Source: CAD feature listing. Evaluate the final solid. Frame: model axes, mm. Face numbers are marked on the shaded views. A direction names the side the tool comes from. Give positions to 0.01 mm unless a question says otherwise; leave off trailing zeros.
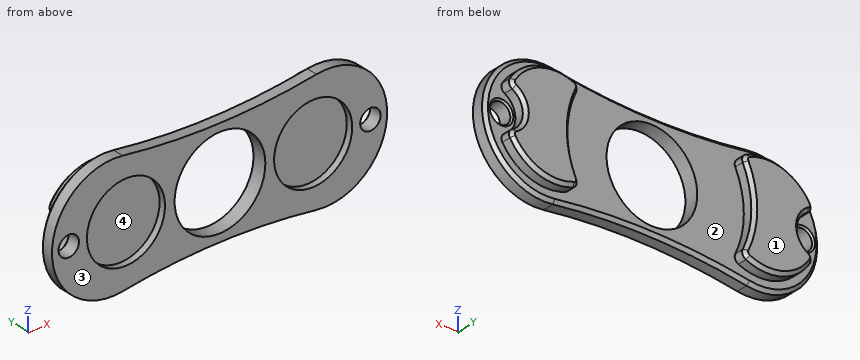
from build123d import *

# Parameters (mm, degrees)
F0_R      = 11.1
F1_DEPTH  = 7
F2_SIZE   = 0.8
F3_R      = 12.5
F4_DEPTH  = 3
F5_R      = 12.5
F6_DEPTH  = 3
F8_R      = 22.5
F9_DEPTH  = 3
F10_R     = 22.5
F11_DEPTH = 3
F12_R     = 5
F13_DEPTH = 3
F14_R     = 5
F15_DEPTH = 3
F16_R     = 5
F17_DEPTH = 3
F18_R     = 5
F19_DEPTH = 3
F20_R     = 1.5
F21_R     = 2.5
F22_DEPTH = 25
F23_R     = 2.5
F24_DEPTH = 25
F25_SIZE  = 0.4
F26_SIZE  = 0.8
F27_W     = 103.2572649419
F27_H     = 49.3412911892
F28_DEPTH = 6.5
F29_R     = 9.55
F30_DEPTH = 1.6


with BuildPart() as f1:
    # F0 (on Front) → F1 (new body)
    with BuildSketch(Plane.XZ):
        with BuildLine():
            ThreePointArc((21.7678643686, 14.8235294118), (-1.9380179843, 13), (-25.6439003372, 14.8235294118))
            ThreePointArc((-25.6439003372, 14.8235294118), (-42.9380179843, 0), (-25.6439003372, -14.8235294118))
            ThreePointArc((-25.6439003372, -14.8235294118), (-1.9380179843, -13), (21.7678643686, -14.8235294118))
            ThreePointArc((21.7678643686, -14.8235294118), (39.0619820157, 0), (21.7678643686, 14.8235294118))
        make_face()
        with Locations((-1.8380179843, 0)):
            Circle(F0_R, mode=Mode.SUBTRACT)
    extrude(amount=F1_DEPTH)

    # F2
    f2_edges = [f1.edges().sort_by_distance(p)[0] for p in [
        (-42.938018, -7, 0),
        (-1.938018, -7, -13),
        (-1.938018, 0, -13),
    ]]
    chamfer(f2_edges, length=F2_SIZE)

    # F3 (on face) → F4 (join)
    with BuildSketch(Plane.XZ.offset(7)):
        with Locations((-27.9380179843, 0)):
            Circle(F3_R)
        with Locations((24.0619820157, 0)):
            Circle(F3_R)
    extrude(amount=F4_DEPTH)

    # F5 (on face) → F6 (join)
    with BuildSketch(Plane(origin=(0, 0, 0), x_dir=(-1, 0, 0), z_dir=(0, 1, 0))):
        with Locations((-24.0619820157, 0)):
            Circle(F5_R)
        with Locations((27.9380179843, 0)):
            Circle(F5_R)
    extrude(amount=F6_DEPTH)

    # F8 (on face) → F9 (cut)
    with BuildSketch(Plane.XZ.offset(10)):
        with Locations((-1.8380179843, 0)):
            Circle(F8_R)
    extrude(amount=-F9_DEPTH, mode=Mode.SUBTRACT)

    # F10 (on face) → F11 (cut)
    with BuildSketch(Plane(origin=(0, 3, 0), x_dir=(-1, 0, 0), z_dir=(0, 1, 0))):
        with Locations((1.8380179843, 0)):
            Circle(F10_R)
    extrude(amount=-F11_DEPTH, mode=Mode.SUBTRACT)

    # F12 (on face) → F13 (cut)
    with BuildSketch(Plane(origin=(0, 3, 0), x_dir=(-1, 0, 0), z_dir=(0, 1, 0))):
        with Locations((-36.5619820157, 0)):
            Circle(F12_R)
    extrude(amount=-F13_DEPTH, mode=Mode.SUBTRACT)

    # F14 (on face) → F15 (cut)
    with BuildSketch(Plane(origin=(0, 3, 0), x_dir=(-1, 0, 0), z_dir=(0, 1, 0))):
        with Locations((40.4380179843, 0)):
            Circle(F14_R)
    extrude(amount=-F15_DEPTH, mode=Mode.SUBTRACT)

    # F16 (on face) → F17 (cut)
    with BuildSketch(Plane.XZ.offset(10)):
        with Locations((-40.4380179843, 0)):
            Circle(F16_R)
    extrude(amount=-F17_DEPTH, mode=Mode.SUBTRACT)

    # F18 (on face) → F19 (cut)
    with BuildSketch(Plane.XZ.offset(10)):
        with Locations((36.5617908537, 0)):
            Circle(F18_R)
    extrude(amount=-F19_DEPTH, mode=Mode.SUBTRACT)

    # F20
    f20_edges = [f1.edges().sort_by_distance(p)[0] for p in [
        (-39.438018, -8.5, 4.898979),
        (-39.438018, -8.5, -4.898979),
        (-21.592999, -8.5, -10.769899),
        (-21.592999, -8.5, 10.769899),
        (17.868739, -8.5, 10.857888),
        (17.868739, -8.5, -10.857888),
        (35.561967, -8.5, -4.899015),
        (35.561967, -8.5, 4.899015),
        (-21.592999, 1.5, -10.769899),
        (-21.592999, 1.5, 10.769899),
        (-39.438018, 1.5, 4.898979),
        (-39.438018, 1.5, -4.898979),
        (17.868739, 1.5, -10.857888),
        (17.868739, 1.5, 10.857888),
        (35.561982, 1.5, -4.898979),
        (35.561982, 1.5, 4.898979),
    ]]
    fillet(f20_edges, radius=F20_R)

    # F21 (on face) → F22 (cut)
    with BuildSketch(Plane.XZ.offset(7)):
        with Locations((-38.8380179843, 0)):
            Circle(F21_R)
    extrude(amount=-F22_DEPTH, mode=Mode.SUBTRACT)

    # F23 (on face) → F24 (cut)
    with BuildSketch(Plane.XZ.offset(7)):
        with Locations((34.9617908537, 0)):
            Circle(F23_R)
    extrude(amount=-F24_DEPTH, mode=Mode.SUBTRACT)

    # F25
    f25_edges = [f1.edges().sort_by_distance(p)[0] for p in [
        (-41.338018, -7, 0),
        (32.461791, -7, 0),
        (32.461791, 0, 0),
        (-41.338018, 0, 0),
    ]]
    chamfer(f25_edges, length=F25_SIZE)

    # F26
    f26_edges = [f1.edges().sort_by_distance(p)[0] for p in [
        (27.97166, -10, 11.872844),
        (18.498441, -10, 10.725925),
        (34.910055, -10, 5.322137),
        (20.661982, -10, 0),
        (31.561791, -10, 0),
        (18.498441, -10, -10.725925),
        (34.910055, -10, -5.322137),
        (27.97166, -10, -11.872844),
        (-24.338018, -10, 0),
        (-22.203581, -10, 10.646558),
        (-22.203581, -10, -10.646558),
        (-31.749718, -10, 11.904661),
        (-31.749718, -10, -11.904661),
        (-38.786142, -10, 5.322071),
        (-38.786142, -10, -5.322071),
        (-35.438018, -10, 0),
        (-24.338018, 3, 0),
        (-22.203581, 3, -10.646558),
        (-22.203581, 3, 10.646558),
        (-31.749718, 3, -11.904661),
        (-31.749718, 3, 11.904661),
        (-38.786142, 3, -5.322071),
        (-38.786142, 3, 5.322071),
        (-35.438018, 3, 0),
        (20.661982, 3, 0),
        (18.498441, 3, 10.725925),
        (18.498441, 3, -10.725925),
        (27.971709, 3, 11.872828),
        (27.971709, 3, -11.872828),
        (34.910106, 3, 5.322071),
        (34.910106, 3, -5.322071),
        (31.561982, 3, 0),
    ]]
    chamfer(f26_edges, length=F26_SIZE)

    # F27 (on face) → F28 (cut)
    with BuildSketch(Plane.XZ.offset(10)):
        with Locations((-3.2676365227, 0)):
            Rectangle(F27_W, F27_H)
    extrude(amount=-F28_DEPTH, mode=Mode.SUBTRACT)

    # F29 (on face) → F30 (cut)
    with BuildSketch(Plane.XZ.offset(3.5)):
        with Locations((-24.8380179843, 0)):
            Circle(F29_R)
        with Locations((20.9617908537, 0)):
            Circle(F29_R)
    extrude(amount=-F30_DEPTH, mode=Mode.SUBTRACT)


solid = f1.part
1) Reachability of the marked faces 3 and 4 from +Z, -Z, +X, -X, +Y, -Y: full face, straight path, thin tool, end or side. Return the list, or none.
Checks:
face 3: +Z, -Z, +X, -X, -Y
face 4: -Y
2) Pull-direction query (X, two-part tool) for the marked faces 1 and 2; classes: +X half, -X half, draft (parallel to the pull), parting line (faces both ways), or undercut.
Checks:
face 1: draft
face 2: undercut
3) First-contact query: pin 1 Ø1.5 at (x, z) = (-21, 7) entering from -Y; pin 2 Ø4.5 at (x, z) = (34.96, 0) entering from -Y; pin 3 Ø1.5 at (y, z) = (-2.5, 12) entering from -X; pin 4 Ø14 at (x, z) = (-14.5, 2) entering from +Y. Flat tips, straight axial feed; report the tip coordinate or a pass-through.
Checks:
pin 1: stops at y = -1.9
pin 2: passes through
pin 3: stops at x = -37.86
pin 4: stops at y = 0
4) Section query A-A on z = 0. State how many separate pieces and enclosed holes the cut face has, and give its area (3 significant figures).
Checks:
separate pieces: 4
enclosed holes: 0
area: 177 mm2
5) Ray query, L1, parallel to X at y = -2, z = 7; L2, parallel to Y at x = -13, z = 7; L3, parallel to Y at x = 28.5, z = -4. Return the intervals inside material, ascending.
Checks:
L1: x = -41.2 to -31.33, -18.34 to -10.45, 6.78 to 14.47, 27.46 to 37.33
L2: y = -3.5 to 0
L3: y = -1.9 to 3
